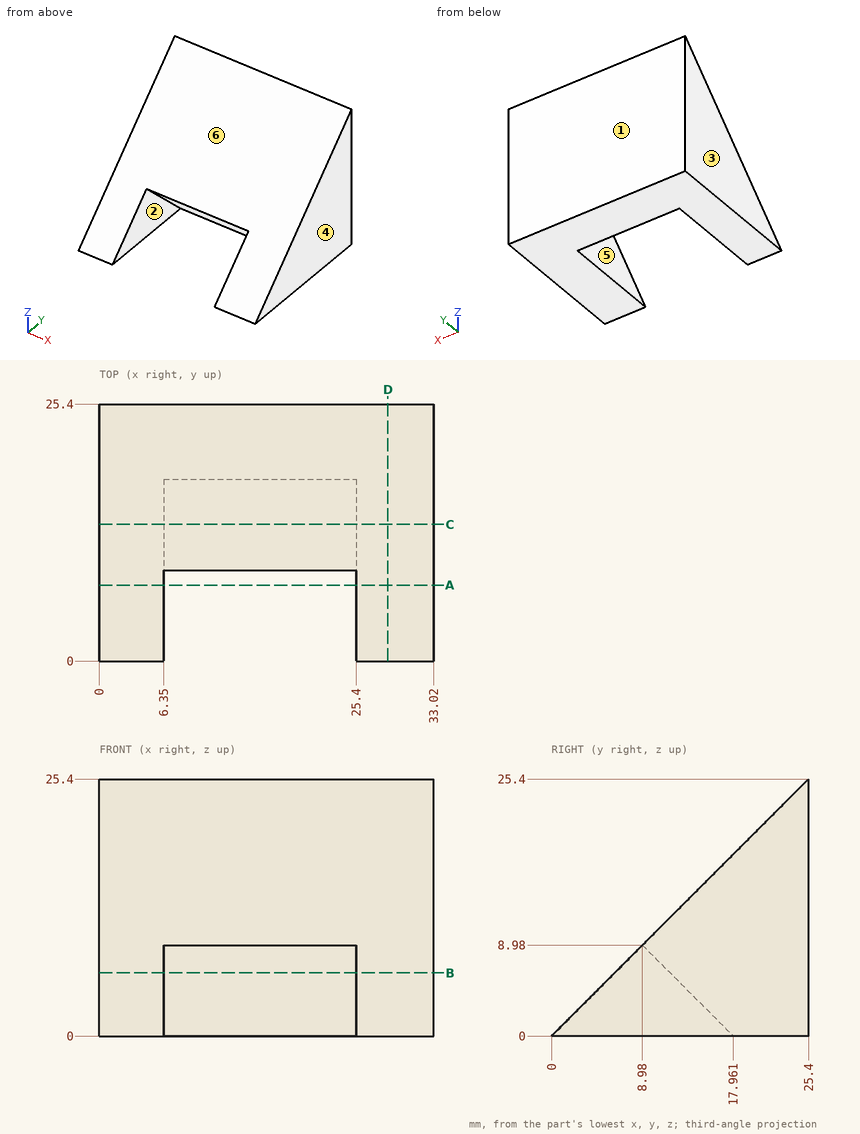
Design review of the part shown in the three views and the two pictorial views. Dimensions are in mm from the part's minimum x, y and z. A direction names the side the tool comes from. Round coordinates to 2 decimals unless told otherwise and drop trailing zeros. Write each loop counter-clockwise with the first axis right and the second up, starting at its lowest first coordinate (ties: lowest second). Pieces come first, ordered by that corner, then holes. Notation, with made-up numbers: (67, 68) - (104, 68) arc R22 ccw to (104, 85) - close; hole circle Ø6 at (63, -18). An arc over 180 degrees is marked (long way). Return JSON: item names as keys, results as strings. Group by question number.
Item 1: We need section C-C on y = 13.5. Write out the cut boundary in (x, z).
Item 2: We need section A-A on y = 7.5. Write out the cut boundary in (x, z), and give its area (3 significant figures).
Item 3: We need section B-B on z = 6.25. Write out the cut boundary in (x, y), and give its area (3 significant figures).
Item 4: We need section D-D on x = 28.5. Write out the cut boundary in (y, z).
Item 5: For probe 1 along X at (y, z) = (11.75, 2); probe 2 along Z at (x, y) = (10.5, 11.5); probe 3 along Y at (x, z) = (10, 3.75), list the stretches that pass through material, from the lowest coordinate up. Write a range as [from, to].
Item 6: Machinability: for the marked faces 1 and 2, which of the approach directions +Z, -Z, +X, -X, +Y, -Y give a long, thin tool a straight path to every point of the face, cutting with its end or side? Answer none if there is none.
Item 7: Insertion check: P1, Ø5, axis at x = 5.5, z = 11.5, coming from the -Y side; P2, Ø12, axis at x = 7.5, z = 19, coming from the -Y side; P3, Ø2, axis at x = 13, z = 5.5, coming from the -Y side. Each pin has a flat end and moves straight along its axis. Give the tip position at first contact, or say it passes through.
Item 8: The part is to be moulded in two halves that separate along X. For the marked faces 3, 4, 5 and 6, say which applies: pulls with the +X half, pulls with the -X half, needs draft (parallel to the pull), parting line crosses it, or undercut.
Model answer:
{
 "1": {"outline": "(0, 0) - (6.35, 0) - (6.35, 4.46) - (25.4, 4.46) - (25.4, 0) - (33.02, 0) - (33.02, 13.5) - (0, 13.5) - close"},
 "2": {"outline": "(0, 0) - (6.35, 0) - (6.35, 7.5) - (0, 7.5) - close; (25.4, 0) - (33.02, 0) - (33.02, 7.5) - (25.4, 7.5) - close", "area": "105 mm²"},
 "3": {"outline": "(0, 6.25) - (6.35, 6.25) - (6.35, 11.71) - (25.4, 11.71) - (25.4, 6.25) - (33.02, 6.25) - (33.02, 25.4) - (0, 25.4) - close", "area": "528 mm²"},
 "4": {"outline": "(0, 0) - (25.4, 0) - (25.4, 25.4) - close"},
 "5": {"probe 1": "x = [0, 6.35], [25.4, 33.02]", "probe 2": "z = [6.46, 11.5]", "probe 3": "y = [14.21, 25.4]"},
 "6": {"face 1": "+Z, -Z, +X, -X, +Y", "face 2": "-Z, -Y"},
 "7": {"P1": "stops at y = 9", "P2": "stops at y = 13", "P3": "stops at y = 11.46"},
 "8": {"face 3": "pulls with the -X half", "face 4": "pulls with the +X half", "face 5": "undercut", "face 6": "needs draft"}
}
